Source: CAD feature listing. Evaluate the final solid. Frame: model axes, mm. A direction names the side the tool comes from. Give positions to 0.01 mm unless a question says otherwise; leave off trailing zeros. Loops run counter-clockwise (first coordinate to the right, second up) from the corner with the lowest first, then second, coordinate; pieces in that order, holes last.
from build123d import *

# Parameters (mm, degrees)
CYLINDER007_R         = 4.8
CYLINDER007_DEPTH     = 15
BOX007_W              = 11
BOX007_H              = 7
BOX007_DEPTH          = 10
FILLET_R              = 3
ARRAY_COUNT           = 2
ARRAY_ANGLE           = 180
ARRAY_PLACEMENT_ANGLE = 90
CYLINDER004_R         = 3
CYLINDER004_DEPTH     = 30
CYLINDER_R            = 3.5
CYLINDER_DEPTH        = 15
CYLINDER006_R         = 4.5
CYLINDER006_DEPTH     = 4
CYLINDER005_R         = 4.5
CYLINDER005_DEPTH     = 4
BOX001_W              = 5
BOX001_H              = 10
BOX001_DEPTH          = 5
BOX002_W              = 20
BOX002_H              = 25
BOX002_DEPTH          = 5
BOX_W                 = 20
BOX_H                 = 5
BOX_DEPTH             = 20
CHAMFER_SIZE          = 0.25
CHAMFER001_SIZE       = 0.25
CHAMFER002_SIZE       = 0.25
FILLET001_R           = 9.9
FILLET002_R           = 2


with BuildPart() as cilindro005:
    # Cylinder007 → Cylinder007 (new body)
    with BuildSketch(Plane.XZ.offset(-23)):
        Circle(CYLINDER007_R)
    extrude(amount=CYLINDER007_DEPTH)


with BuildPart() as array:
    # Box007 → Box007 (new body)
    with BuildSketch(Plane(origin=(10, 5, -5), x_dir=(1, 0, 0), z_dir=(0, 0, 1))):
        with Locations((5.5, 3.5)):
            Rectangle(BOX007_W, BOX007_H)
    extrude(amount=BOX007_DEPTH)


with BuildPart() as array_1:
    # BaseFeature placement: moved
    add(array.part.moved(Location((-10, -5, 5))))

    # Fillet
    fillet_edges = [array_1.edges().sort_by_distance(p)[0] for p in [
        (5.5, 0, 10),
        (5.5, 0, 0),
    ]]
    fillet(fillet_edges, radius=FILLET_R)


with BuildPart() as array_2:
    # Body placement: moved
    add(array_1.part.moved(Location((-5, 5, 0))))

    # Array: Array ×2 about axis
    array_axis = Axis((0, 0, 0), (0, 0, 1))


with BuildPart() as array_3:
    add(array_2.part)
    for i in range(1, ARRAY_COUNT):
        add(array_2.part.rotate(array_axis, i * ARRAY_ANGLE / (ARRAY_COUNT - 1)))


with BuildPart() as array_4:
    # Array placement: moved
    add(array_3.part.moved(Location((0, -3, -5))).rotate(Axis((0, -3, -5), (0, 0, 1)), ARRAY_PLACEMENT_ANGLE))


with BuildPart() as cilindro004:
    # Cylinder004 → Cylinder004 (new body)
    with BuildSketch(Plane(origin=(0, 15, -15), x_dir=(1, 0, 0), z_dir=(0, 0, 1))):
        Circle(CYLINDER004_R)
    extrude(amount=CYLINDER004_DEPTH)


with BuildPart() as cilindro:
    # Cylinder → Cylinder (new body)
    with BuildSketch(Plane.XZ.offset(-5)):
        Circle(CYLINDER_R)
    extrude(amount=CYLINDER_DEPTH)


with BuildPart() as obj1:
    # Cylinder006 → Cylinder006 (new body)
    with BuildSketch(Plane.XY.offset(4.3)):
        Circle(CYLINDER006_R)
    extrude(amount=CYLINDER006_DEPTH)


with BuildPart() as fusion003:
    # Cylinder005 → Cylinder005 (new body)
    with BuildSketch(Plane.XY.offset(-8.3)):
        Circle(CYLINDER005_R)
    extrude(amount=CYLINDER005_DEPTH)

    # Fusion003: union obj1
    add(obj1.part)


with BuildPart() as fusion003_1:
    # Fusion003 placement: moved
    add(fusion003.part.moved(Location((0, 15, 0))))


with BuildPart() as pin0:
    # Box001 → Box001 (new body)
    with BuildSketch(Plane(origin=(-2.5, -10, 5), x_dir=(1, 0, 0), z_dir=(0, 0, 1))):
        with Locations((2.5, 5)):
            Rectangle(BOX001_W, BOX001_H)
    extrude(amount=BOX001_DEPTH)


with BuildPart() as pin001:
    # Clone base: copy of pin0
    add(pin0.part)


with BuildPart() as pin001_1:
    # Clone placement: moved
    add(pin001.part.moved(Location((0, 0, -15))))


with BuildPart() as pared1:
    # Box002 → Box002 (new body)
    with BuildSketch(Plane(origin=(-10, 0, 5), x_dir=(1, 0, 0), z_dir=(0, 0, 1))):
        with Locations((10, 12.5)):
            Rectangle(BOX002_W, BOX002_H)
    extrude(amount=BOX002_DEPTH)


with BuildPart() as pared002:
    # Clone001 base: copy of pared1
    add(pared1.part)


with BuildPart() as pared002_1:
    # Clone001 placement: moved
    add(pared002.part.moved(Location((0, 0, -15))))


with BuildPart() as fillet002:
    # Box → Box (new body)
    with BuildSketch(Plane(origin=(-10, -5, -10), x_dir=(1, 0, 0), z_dir=(0, 0, 1))):
        with Locations((10, 2.5)):
            Rectangle(BOX_W, BOX_H)
    extrude(amount=BOX_DEPTH)

    # Fusion: union pin0, pin001, pared1, pared002
    add(pin0.part)
    add(pin001_1.part)
    add(pared1.part)
    add(pared002_1.part)

    # Fusion004: union Fusion003
    add(fusion003_1.part)

    # Cut001: cut Cilindro
    add(cilindro.part, mode=Mode.SUBTRACT)

    # Cut002: cut Cilindro004
    add(cilindro004.part, mode=Mode.SUBTRACT)

    # Cut003: cut Array
    add(array_4.part, mode=Mode.SUBTRACT)

    # Cut004: cut Cilindro005
    add(cilindro005.part, mode=Mode.SUBTRACT)

    # Chamfer
    chamfer_edges = [fillet002.edges().sort_by_distance(p)[0] for p in [
        (3.863213, 17.307723, 4.3),
        (3.863213, 12.692277, 4.3),
    ]]
    chamfer(chamfer_edges, length=CHAMFER_SIZE)

    # Chamfer001
    chamfer001_edges = [fillet002.edges().sort_by_distance(p)[0] for p in [
        (-4.5, 15, 4.3),
    ]]
    chamfer(chamfer001_edges, length=CHAMFER001_SIZE)

    # Chamfer002
    chamfer002_edges = [fillet002.edges().sort_by_distance(p)[0] for p in [
        (3.863213, 17.307723, -4.3),
        (-4.5, 15, -4.3),
        (3.863213, 12.692277, -4.3),
    ]]
    chamfer(chamfer002_edges, length=CHAMFER002_SIZE)

    # Fillet001
    fillet001_edges = [fillet002.edges().sort_by_distance(p)[0] for p in [
        (-10, 25, -7.5),
        (10, 25, -7.5),
        (-10, 25, 7.5),
        (10, 25, 7.5),
    ]]
    fillet(fillet001_edges, radius=FILLET001_R)

    # Fillet002
    fillet002_edges = [fillet002.edges().sort_by_distance(p)[0] for p in [
        (-10, 5.05, -10),
        (-10, 5.05, 10),
    ]]
    fillet(fillet002_edges, radius=FILLET002_R)


solid = fillet002.part
1) Ray query, probe 1 along Z at (x, y) = (-3.75, 21); probe 2 along Z at (x, y) = (0, -2.65); probe 3 along X at (y, z) = (-2.5, 0). Return the intervals inside material, ascending.
Checks:
probe 1: z = -10 to -5, 5 to 10
probe 2: z = -10 to -3.5, 3.5 to 10
probe 3: x = -5 to -3.5, 3.5 to 5
2) Cut plane C-C (y = -3). Return loops of the section in (x, z), and give its area (3 significant figures).
Checks:
outline: (-10, -8) arc R2 ccw to (-8, -10) - (8, -10) arc R2 ccw to (10, -8) - (10, -5) - (8, -5) arc R3 cw to (5, -2) - (5, 2) arc R3 cw to (8, 5) - (10, 5) - (10, 8) arc R2 ccw to (8, 10) - (-8, 10) arc R2 ccw to (-10, 8) - (-10, 5) - (-8, 5) arc R3 cw to (-5, 2) - (-5, -2) arc R3 cw to (-8, -5) - (-10, -5) - close; hole circle Ø7 at (0, 0)
area: 266 mm2
3) Contact query for flat-ended pins moving along their axis: P1, Ø10, axis at x = -4.5, z = 1.5, coming from the +Y side; P2, Ø5, axis at x = -3.5, z = -1.5, coming from the +Y side; P3, Ø3.5, axis at x = 0, y = 15, coming from the +Z side; P4, Ø1, axis at x = -5, z = 8, coming from the +Y side. Output: stop coordinate, or through.
Checks:
P1: stops at y = 24.97
P2: stops at y = 0
P3: passes through
P4: stops at y = 23.97
4) Pull-direction query (Z, two-part tool) for faces 1 (the cylindrical face through (-9.4, 4.91, -9.43)), 2 (the cylindrical face through (0, 18, 7)), 3 (the cylindrical face through (4.16, 13.28, -4.78)); classes: released by +Z, released by -Z, zero draft, split by the parting line, or undercut.
Checks:
face 1: released by -Z
face 2: zero draft
face 3: undercut
5) Cut plane D-D (z = -7.25). Return loops of the section in (x, y).
Checks:
outline: (-10, -5) - (-2.5, -5) - (-2.5, -10) - (2.5, -10) - (2.5, -5) - (10, -5) - (10, 15.1) arc R9.9 ccw to (0.1, 25) - (-0.1, 25) arc R9.9 ccw to (-10, 15.1) - close; hole circle Ø6 at (0, 15)
6) Cut plane A-A (y = 2). Return loops of the section in (x, z).
Checks:
outline: (-10, -8) arc R2 ccw to (-8, -10) - (8, -10) arc R2 ccw to (10, -8) - (10, -5) - (-10, -5) - close; (-10, 5) - (10, 5) - (10, 8) arc R2 ccw to (8, 10) - (-8, 10) arc R2 ccw to (-10, 8) - close
7) Cut plane B-B (z = 0). Return loops of the section in (x, y), and give its area (3 significant figures).
Checks:
outline: (-5, -5) - (-3.5, -5) - (-3.5, 0) - (-5, 0) - close; (3.5, -5) - (5, -5) - (5, 0) - (3.5, 0) - close
area: 15.0 mm2
8) Reachability of faces 4 (the cylindrical face through (0, 11.4, -4.8)), 5 (the flat face through (-3.2, 15.1, -4.3)), 6 (the cylindrical face through (4.16, 13.28, 4.77)) from +Z, -Z, +X, -X, +Y, -Y: full face, straight path, thin tool, end or side. Return the list, or none.
Checks:
face 4: +Y
face 5: +X, -X, +Y
face 6: none
